from build123d import *
from build123d.topology import SkipClean

# Parameters (mm, degrees)
SKETCH1_R           = 5
BOSS_EXTRUDE1_DEPTH = 1.5875
SKETCH2_R           = 50
SKETCH2_R_2         = 45
BOSS_EXTRUDE2_DEPTH = 341.625
SKETCH3_R           = 5
BOSS_EXTRUDE3_DEPTH = 0.218965517
BOSS_EXTRUDE4_START = 20
SKETCH4_R           = 5
BOSS_EXTRUDE4_DEPTH = 20
BOSS_EXTRUDE5_START = 20
SKETCH5_R           = 5
BOSS_EXTRUDE5_DEPTH = 20


with BuildPart() as part:
    # Sketch1 → Boss-Extrude1 (new body)
    with BuildSketch(Plane(origin=(0, 0, 0), x_dir=(1, 0, 0), z_dir=(0, 1, 0))):
        with BuildLine():
            Line((-395, 50), (395, 50))
            ThreePointArc((395, 50), (416.213203436, 41.213203436), (425, 20))
            Line((425, 20), (425, -20))
            ThreePointArc((425, -20), (416.213203436, -41.213203436), (395, -50))
            Line((395, -50), (-395, -50))
            ThreePointArc((-395, -50), (-416.213203436, -41.213203436), (-425, -20))
            Line((-425, -20), (-425, 20))
            ThreePointArc((-425, 20), (-416.213203436, 41.213203436), (-395, 50))
        make_face()
        with Locations(Location((-395, 20, 0), (0, 0, 270))):
            Circle(SKETCH1_R, mode=Mode.SUBTRACT)
        with Locations(Location((-395, -20, 0), (0, 0, 270))):
            Circle(SKETCH1_R, mode=Mode.SUBTRACT)
        with Locations(Location((395, 20, 0), (0, 0, 270))):
            Circle(SKETCH1_R, mode=Mode.SUBTRACT)
        with Locations(Location((395, -20, 0), (0, 0, 270))):
            Circle(SKETCH1_R, mode=Mode.SUBTRACT)
    extrude(amount=BOSS_EXTRUDE1_DEPTH)

    # Sketch2 → Boss-Extrude2 (add)
    with BuildSketch(Plane.XZ):
        with Locations(Location((0, 0, 0), (0, 0, 270))):
            Circle(SKETCH2_R)
        with Locations(Location((0, 0, 0), (0, 0, 270))):
            Circle(SKETCH2_R_2, mode=Mode.SUBTRACT)
    extrude(amount=BOSS_EXTRUDE2_DEPTH)

    # Sketch3 → Boss-Extrude3 (add)
    with BuildSketch(Plane.XZ.offset(341.625)):
        with BuildLine():
            Line((-130, 50), (130, 50))
            ThreePointArc((130, 50), (144.142135624, 44.142135624), (150, 30))
            Line((150, 30), (150, -30))
            ThreePointArc((150, -30), (144.142135624, -44.142135624), (130, -50))
            Line((130, -50), (-130, -50))
            ThreePointArc((-130, -50), (-144.142135624, -44.142135624), (-150, -30))
            Line((-150, -30), (-150, 30))
            ThreePointArc((-150, 30), (-144.142135624, 44.142135624), (-130, 50))
        make_face()
        with Locations(Location((-130, 30, 0), (0, 0, 270))):
            Circle(SKETCH3_R, mode=Mode.SUBTRACT)
        with Locations(Location((-130, -30, 0), (0, 0, 270))):
            Circle(SKETCH3_R, mode=Mode.SUBTRACT)
        with Locations(Location((130, 30, 0), (0, 0, 270))):
            Circle(SKETCH3_R, mode=Mode.SUBTRACT)
        with Locations(Location((130, -30, 0), (0, 0, 270))):
            Circle(SKETCH3_R, mode=Mode.SUBTRACT)
    extrude(amount=BOSS_EXTRUDE3_DEPTH)

    # Sketch4 → Boss-Extrude4 (add)
    # profile 1 of 2: a face of its own
    with SkipClean():  # the faces are left unmerged after this step: merging them gives an invalid solid
        with BuildSketch(Plane.XZ.offset(BOSS_EXTRUDE4_START)):
            with BuildLine():
                ThreePointArc((0, 50), (50, 0), (0, -50))
                Line((0, -50), (395, -50))
                ThreePointArc((395, -50), (416.213203436, -41.213203436), (425, -20))
                Line((425, -20), (425, 20))
                ThreePointArc((425, 20), (416.213203436, 41.213203436), (395, 50))
                Line((395, 50), (0, 50))
            make_face()
            with Locations((395, -20)):
                Circle(SKETCH4_R, mode=Mode.SUBTRACT)
            with Locations((395, 20)):
                Circle(SKETCH4_R, mode=Mode.SUBTRACT)
        # profile 2 of 2: a face of its own
        with BuildSketch(Plane.XZ.offset(BOSS_EXTRUDE4_START)):
            with BuildLine():
                Line((-395, -50), (0, -50))
                ThreePointArc((0, -50), (-50, 0), (0, 50))
                Line((0, 50), (-395, 50))
                ThreePointArc((-395, 50), (-416.213203436, 41.213203436), (-425, 20))
                Line((-425, 20), (-425, -20))
                ThreePointArc((-425, -20), (-416.213203436, -41.213203436), (-395, -50))
            make_face()
            with Locations((-395, -20)):
                Circle(SKETCH4_R, mode=Mode.SUBTRACT)
            with Locations((-395, 20)):
                Circle(SKETCH4_R, mode=Mode.SUBTRACT)
        extrude(amount=-BOSS_EXTRUDE4_DEPTH)

    # Sketch5 → Boss-Extrude5 (add)
    # profile 1 of 2: a face of its own
    with SkipClean():  # the faces are left unmerged after this step: merging them gives an invalid solid
        with BuildSketch(Plane(origin=(0, -341.625, 0), x_dir=(1, 0, 0), z_dir=(0, 1, 0)).offset(BOSS_EXTRUDE5_START)):
            with BuildLine():
                ThreePointArc((150, 30), (144.142135624, 44.142135624), (130, 50))
                Line((130, 50), (0, 50))
                ThreePointArc((0, 50), (50, 0), (0, -50))
                Line((0, -50), (130, -50))
                ThreePointArc((130, -50), (144.142135624, -44.142135624), (150, -30))
                Line((150, -30), (150, 30))
            make_face()
            with Locations((130, -30)):
                Circle(SKETCH5_R, mode=Mode.SUBTRACT)
            with Locations((130, 30)):
                Circle(SKETCH5_R, mode=Mode.SUBTRACT)
        # profile 2 of 2: a face of its own
        with BuildSketch(Plane(origin=(0, -341.625, 0), x_dir=(1, 0, 0), z_dir=(0, 1, 0)).offset(BOSS_EXTRUDE5_START)):
            with BuildLine():
                ThreePointArc((0, -50), (-50, 0), (0, 50))
                Line((0, 50), (-130, 50))
                ThreePointArc((-130, 50), (-144.142135624, 44.142135624), (-150, 30))
                Line((-150, 30), (-150, -30))
                ThreePointArc((-150, -30), (-144.142135624, -44.142135624), (-130, -50))
                Line((-130, -50), (0, -50))
            make_face()
            with Locations((-130, -30)):
                Circle(SKETCH5_R, mode=Mode.SUBTRACT)
            with Locations((-130, 30)):
                Circle(SKETCH5_R, mode=Mode.SUBTRACT)
        extrude(amount=-BOSS_EXTRUDE5_DEPTH)


solid = part.part
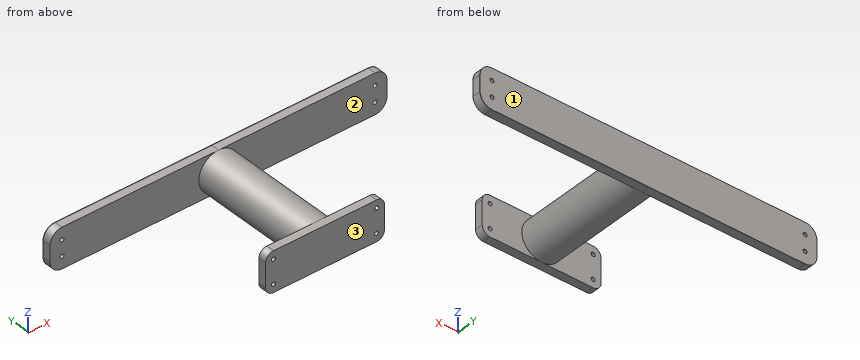
Model file for the job. Use its own axes, mm. Face numbers are marked on the shaded views. Round coordinates to 2 decimals unless told otherwise and drop trailing zeros. Loops run counter-clockwise (first coordinate to the right, second up) from the corner with the lowest first, then second, coordinate; pieces in that order, holes last. Notation, with made-up numbers: M -22,73 L -7,73 A14 ccw -7,88 Z; hole C 31,-32.75 d1. An arc over 180 degrees is marked long. One line per question, with ' | ' between items.
1) Flat gauge pins, fed straight in: pin 1 (8 mm diameter, centred on x = 130, z = -30, fed in from -Y); pin 2 (8 mm diameter, centred on x = -395, z = -20, fed in from +Y); pin 3 (2 mm diameter, centred on y = -305, z = 37, fed in from +X). Where does each tip first touch, or does it go through?
Solved:
pin 1: stops at y = -20 | pin 2: passes through | pin 3: stops at x = 34.7
2) Drill centre lines: line 1 along Z through (x, y) = (-395, 1.25); line 2 along X through (y, z) = (1, 20); line 3 along Y through (x, z) = (112.5, 41) (1 decimal). Where is each one in solid material? Low to high.
Solved:
line 1: z = -50 to -25, -15 to 15, 25 to 50 | line 2: x = -425 to -400, -390 to 390, 400 to 425 | line 3: y = -341.8 to -321.6, -20 to 1.6
3) Mould opens along Y. For the marked faces 1, 2 and 3 say: +Y half, -Y half, draft (parallel to the pull), parting line (faces both ways), or undercut.
Solved:
face 1: +Y half | face 2: undercut | face 3: -Y half
4) Band-saw the part on B-B (x = -247). Give the cut face in (y, z).
Solved:
outline: M -20,-50 L 1.59,-50 L 1.59,50 L -20,50 Z
5) Band-saw the part on C-C (y = -220). Give the cut face in (x, z).
Solved:
outline: C 0,0 d100; hole C 0,0 d90
6) Band-saw the part on A-A (z = -1). Give the cut face in (x, y) (1 decimal), then the cut area to 3 significant figures.
Solved:
outline: M -425,-20 L -50,-20 L -50,-321.6 L -150,-321.6 L -150,-341.8 L 150,-341.8 L 150,-321.6 L 50,-321.6 L 50,-20 L 425,-20 L 425,1.6 L -425,1.6 Z; hole M -45,-341.6 L 45,-341.6 L 45,0 L -45,0 Z | area: 23,800 mm²
